The model under review builds one solid part; all positions refer to its coordinate system, in mm. A direction names the side the tool comes from. Round coordinates to 2 decimals unless told otherwise and drop trailing zeros. Write each loop counter-clockwise with the first axis right and the second up, starting at its lowest first coordinate (ties: lowest second). Pieces come first, ordered by that corner, then holes. Notation, with made-up numbers: M 50,39 L 99,39 A21 ccw 99,52 Z; hole C 3.25,-10 d6. An arc over 180 degrees is marked long. Write item = value, one per line. Start each with the question number.
Item 1: Take a section at C-C, the plane y = 1.25. Give the boundary of the cut face in (x, z), plus the area to 3 significant figures.
Item 2: Take a section at B-B, the plane z = 0. Give the boundary of the cut face in (x, y) (3 decimals).
Item 3: The part is to be moulded in two halves that separate along X. For faces 1 (the cylindrical face through (-1.19, 0.82, -5.37)), 2 (the cylindrical face through (1.29, 3.245, 2.024)), 3 (the flat face through (-1, 1.626, 4)), say which applies: +X half, -X half, draft (parallel to the pull), parting line (faces both ways), or undercut.
Item 4: For pin 1 Ø1 at (x, y) = (2, 1) entering from +Z; pin 2 Ø3 at (y, z) = (4, -4) entering from +X, all flat-tipped, find the tip position at first contact; note any pin that passes through.
Item 5: Tool access review of faces 4 (the flat face through (3, 0, -1)), 5 (the cylindrical face through (-2.893, 4.034, 2.653)): name each direction out of +Z, -Z, +X, -X, +Y, -Y from which nothing blocks a thin tool from reaching the whole face with its end or side.
Item 6: To check wall thickness, follow line 1 along Z through (x, y) = (0, 4.5) (3 decimals); line 2 along Z through (x, y) = (-1, 3.25); line 3 along X through (y, z) = (2.5, -1.25). State the ranges of each line that lie inside material, in increasing order.
Item 7: Take a section at A-A, the plane x = 0. Give the boundary of the cut face in (y, z) (3 decimals).
Item 8: Take a section at D-D, the plane x = -5. Give the boundary of the cut face in (y, z).
from build123d import *

# Parameters (mm, degrees)
SKETCH2_W               = 14
SKETCH2_H               = 8
CUT_EXTRUDE1_DEPTH      = 6.5
CUT_EXTRUDE1_DEPTH_BACK = 6.5
CHAMFER1_SIZE           = 0.25


with BuildPart() as part:
    # Sketch1 → Revolve1 (revolve)
    with BuildSketch(Plane.XY):
        Polygon((3.925, 1.6256), (3.925, 12.4), (2.4, 12.4), (2.4, 0.2), (2.6, 0), (5.5, 0), (5.5, 1.6256), align=None)
    revolve(axis=Axis((0, 0, 0), (0, -1, 0)))

    # Sketch2 → Cut-Extrude1 (cut, two sides)
    with BuildSketch(Plane.XY) as cut_extrude1_sk:
        with Locations((0, 10.6256)):
            Rectangle(SKETCH2_W, SKETCH2_H)
    extrude(amount=CUT_EXTRUDE1_DEPTH, mode=Mode.SUBTRACT)
    extrude(cut_extrude1_sk.sketch, amount=-CUT_EXTRUDE1_DEPTH_BACK, mode=Mode.SUBTRACT)

    # Chamfer1
    chamfer1_edges = [part.edges().sort_by_distance(p)[0] for p in [
        (-3.925, 6.6256, 0),
        (-2.4, 6.6256, 0),
    ]]
    chamfer(chamfer1_edges, length=CHAMFER1_SIZE)


solid = part.part
Response values:
q1.outline = C 0,0 d11; hole C 0,0 d4.8
q1.area = 76.9 mm2
q2.outline = M -5.5,0 L -2.6,0 L -2.4,0.2 L -2.4,6.376 L -2.65,6.626 L -3.675,6.626 L -3.925,6.376 L -3.925,1.626 L -5.5,1.626 Z; M 2.4,0.2 L 2.6,0 L 5.5,0 L 5.5,1.626 L 3.925,1.626 L 3.925,6.376 L 3.675,6.626 L 2.65,6.626 L 2.4,6.376 Z
q3.face_1 = parting line
q3.face_2 = undercut
q3.face_3 = draft
q4.pin_1 = 5.29
q4.pin_2 = 3.03
q5.face_4 = +Z, -Z, +X, -X, -Y
q5.face_5 = +Y
q6.line_1 = -3.925 to -2.4, 2.4 to 3.925
q6.line_2 = -3.8 to -2.18, 2.18 to 3.8
q6.line_3 = -3.72 to -2.05, 2.05 to 3.72
q7.outline = M 0,-5.5 L 1.626,-5.5 L 1.626,-3.925 L 6.376,-3.925 L 6.626,-3.675 L 6.626,-2.65 L 6.376,-2.4 L 0.2,-2.4 L 0,-2.6 Z; M 0,2.6 L 0.2,2.4 L 6.376,2.4 L 6.626,2.65 L 6.626,3.675 L 6.376,3.925 L 1.626,3.925 L 1.626,5.5 L 0,5.5 Z
q8.outline = M 0,-2.29 L 1.63,-2.29 L 1.63,2.29 L 0,2.29 Z
